Geometry: final body of the model. Coordinates: model frame, mm. Face numbers are marked on the shaded views. A direction names the side the tool comes from. Give positions to 0.01 mm unless a question says otherwise; leave off trailing zeros.
```python
from build123d import *

# Parameters (mm, degrees)
SKETCH_1_R                = 30.196888946
EXTRUDE_1_DEPTH           = 12
CUT_EXTRUDE_1_DEPTH       = 2.4
SKETCH_3_R                = 1.5
CUT_EXTRUDE_2_DEPTH       = 3.6
SKETCH_6_R                = 2.05
CUT_EXTRUDE_3_DEPTH       = 67.802158421
PATTERN_CIRCULAR_25_COUNT = 8
CHAMFER_1_SIZE            = 3
SKETCH_7_R                = 24.696170665
CUT_EXTRUDE_4_DEPTH       = 1.5
SKETCH_8_R                = 1.6
CUT_EXTRUDE_5_DEPTH       = 44.976746335


with BuildPart() as part:
    # 草图1 → 凸台-拉伸1 (new body)
    with BuildSketch(Plane(origin=(0, 0, 0), x_dir=(1, 0, 0), z_dir=(0, 1, 0))):
        with Locations(Location((0, 0, 0), (0, 0, 270))):
            Circle(SKETCH_1_R)
        Polygon((13.927295841, 13.927295841), (0, 19.696170665), (-13.927295841, 13.927295841), (-19.696170665, 0), (-13.927295841, -13.927295841), (0, -19.696170665), (13.927295841, -13.927295841), (19.696170665, 0), align=None, mode=Mode.SUBTRACT)
    extrude(amount=EXTRUDE_1_DEPTH)

    # 草图2 → 切除-拉伸1 (cut)
    with BuildSketch(Plane(origin=(6.96364792, 0, -16.811733253), x_dir=(0.9238795325112867, 0, 0.38268343236508984), z_dir=(-0.38268343236508984, 0, 0.9238795325112867))):
        Polygon((3.233161507, 6), (1.616580754, 8.8), (-1.616580754, 8.8), (-3.233161507, 6), (-1.616580754, 3.2), (1.616580754, 3.2), align=None)
    cut_extrude_1 = extrude(amount=-CUT_EXTRUDE_1_DEPTH, mode=Mode.SUBTRACT)

    # 草图3 → 切除-拉伸2 (cut)
    with BuildSketch(Plane(origin=(7.882088158, 0, -19.029044131), x_dir=(0.9238795325112867, 0, 0.3826834323650899), z_dir=(-0.3826834323650899, 0, 0.9238795325112867))):
        with Locations((0, 6)):
            Circle(SKETCH_3_R)
    cut_extrude_2 = extrude(amount=-CUT_EXTRUDE_2_DEPTH, mode=Mode.SUBTRACT)

    # 草图6 → 切除-拉伸3 (cut, through all)
    with BuildSketch(Plane(origin=(9.259748515, 0, -22.355010448), x_dir=(0.923879532511287, 0, 0.38268343236508945), z_dir=(-0.38268343236508945, 0, 0.923879532511287))):
        with Locations((0, 6)):
            Circle(SKETCH_6_R)
    cut_extrude_3 = extrude(amount=-CUT_EXTRUDE_3_DEPTH, mode=Mode.SUBTRACT)

    # 阵列(圆周)25: 切除-拉伸1, 切除-拉伸2, 切除-拉伸3 ×8 about axis
    pattern_circular_25_axis = Axis((0, 0, 0), (0, 1, 0))
    add([cut_extrude_1.rotate(pattern_circular_25_axis, i * 360 / PATTERN_CIRCULAR_25_COUNT) for i in range(1, PATTERN_CIRCULAR_25_COUNT)], mode=Mode.SUBTRACT)
    add([cut_extrude_2.rotate(pattern_circular_25_axis, i * 360 / PATTERN_CIRCULAR_25_COUNT) for i in range(1, PATTERN_CIRCULAR_25_COUNT)], mode=Mode.SUBTRACT)
    add([cut_extrude_3.rotate(pattern_circular_25_axis, i * 360 / PATTERN_CIRCULAR_25_COUNT) for i in range(1, PATTERN_CIRCULAR_25_COUNT)], mode=Mode.SUBTRACT)

    # 倒角1
    chamfer_1_edges = [part.edges().sort_by_distance(p)[0] for p in [
        (0, 12, -30.196888946),
    ]]
    chamfer(chamfer_1_edges, length=CHAMFER_1_SIZE)

    # 草图7 → 切除-拉伸4 (cut)
    with BuildSketch(Plane(origin=(0, 12, 0), x_dir=(1, 0, 0), z_dir=(0, 1, 0))):
        with Locations(Location((0, 0, 0), (0, 0, 270))):
            Circle(SKETCH_7_R)
    extrude(amount=-CUT_EXTRUDE_4_DEPTH, mode=Mode.SUBTRACT)

    # 草图8 → 切除-拉伸5 (cut, through all)
    with BuildSketch(Plane(origin=(0, 10.5, 0), x_dir=(1, 0, 0), z_dir=(0, 1, 0))):
        with Locations(Location((0, 22.196170665, 0), (0, 0, 270))):
            Circle(SKETCH_8_R)
        with Locations(Location((15.695062794, 15.695062794, 0), (0, 0, 270))):
            Circle(SKETCH_8_R)
        with Locations(Location((22.196170665, 0, 0), (0, 0, 270))):
            Circle(SKETCH_8_R)
        with Locations(Location((15.695062794, -15.695062794, 0), (0, 0, 270))):
            Circle(SKETCH_8_R)
        with Locations(Location((0, -22.196170665, 0), (0, 0, 270))):
            Circle(SKETCH_8_R)
        with Locations(Location((-15.695062794, -15.695062794, 0), (0, 0, 270))):
            Circle(SKETCH_8_R)
        with Locations(Location((-22.196170665, 0, 0), (0, 0, 270))):
            Circle(SKETCH_8_R)
        with Locations(Location((-15.695062794, 15.695062794, 0), (0, 0, 270))):
            Circle(SKETCH_8_R)
    extrude(amount=-CUT_EXTRUDE_5_DEPTH, mode=Mode.SUBTRACT)


solid = part.part
```
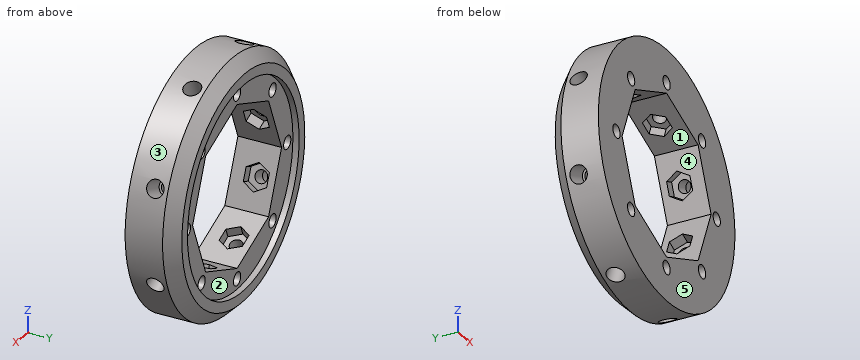
Item 1: Reachability of the marked faces 1 and 2 from +Z, -Z, +X, -X, +Y, -Y: full face, straight path, thin tool, end or side. Return the list, or none.
Found:
face 1: +Y, -Y
face 2: +Y
Item 2: Section A-A, the plane y = 1.25. State how many separate pieces and enclosed holes the cut face has, plus the area to 3 significant figures.
Found:
separate pieces: 1
enclosed holes: 9
area: 1,700 mm2
Item 3: Line query: L1, parallel to X at y = 7.25, z = 0; L2, parallel to X at y = 7.5, z = -27; L3, parallel to X at y = 2.25, z = 14.5. Output: solid intervals per line, ascending.
Found:
L1: x = -30.2 to -23.8, -20.6 to -19.7, 19.7 to 20.6, 23.8 to 30.2
L2: x = -13.52 to -12.7, -9.67 to 9.67, 12.7 to 13.52
L3: x = -26.49 to -16.76, -14.63 to -12.54, 12.54 to 14.63, 16.76 to 26.49
Item 4: Pull-direction query (X, two-part tool) for the marked faces 3, 4 and 5; classes: +X half, -X half, draft (parallel to the pull), parting line (faces both ways), or undercut.
Found:
face 3: parting line
face 4: undercut
face 5: draft
Item 5: Pin query (flat end, axial travel): pin 1 Ø5 at (x, y) = (5, 9) entering from -Z; pin 2 Ø1 at (x, z) = (-17.5, 6.5) entering from +Y; pin 3 Ø1.5 at (x, y) = (-18, 4) entering from +Z. Return the tip coordinate at first contact, or that it passes through.
Found:
pin 1: stops at z = -30.09
pin 2: stops at y = 10.5
pin 3: stops at z = 24.78
